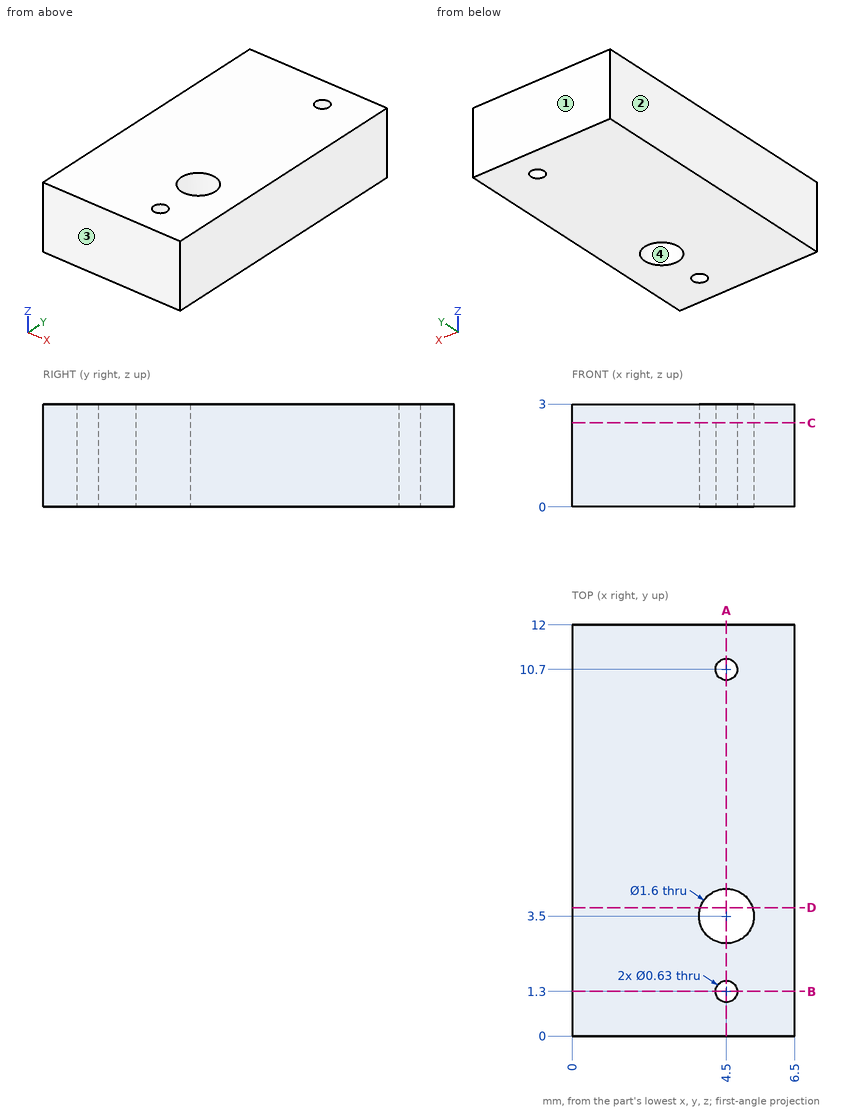
Part print with two shaded views. Sizes in mm from the minimum x, y, z corner. Coordinates: 2 decimals unless noted, no trailing zeros. Write each loop counter-clockwise with the first axis right and the second up, starting at its lowest first coordinate (ties: lowest second). Pieces come first, ordered by that corner, then holes.
(1) Cut at D-D on y = 3.75. List the corners of the cut face in (x, z).
(2) Drill centre lines: line 1 (Y direction, x = 4.5, z = 0.95) (3 decimals); line 2 (X direction, y = 3.5, z = 2.3); line 3 (Y direction, x = 4, z = 1.35). Where is each one in solid material? Low to high.
(3) Pin check, flat tip, straight feed: pin 1 Ø1.5 at (x, y) = (3, 6.5) entering from -Z. Stop position of the tip, or through.
(4) Mould opens along Y. For the marked faces 1, 2, 3 and 4 say: pulls with the +Y half, pulls with the -Y half, needs draft (parallel to the pull), parting line crosses it, or undercut.
(5) Cut at B-B on y = 1.3. List the corners of the cut face in (x, z) (3 decimals).
(6) Cut at C-C on z = 2.45. List the corners of the cut face in (x, y) (3 decimals), and give its area (3 significant figures).
(7) Cut at A-A on x = 4.5. List the corners of the cut face in (y, z) (3 decimals), and give its area (3 significant figures).
Working result:
1. outline: (0, 0) - (3.74, 0) - (3.74, 3) - (0, 3) - close; (5.26, 0) - (6.5, 0) - (6.5, 3) - (5.26, 3) - close
2. line 1: y = 0 to 0.985, 1.615 to 2.7, 4.3 to 10.385, 11.015 to 12
2. line 2: x = 0 to 3.7, 5.3 to 6.5
2. line 3: y = 0 to 2.88, 4.12 to 12
3. pin 1: stops at z = 0
4. face 1: pulls with the +Y half
4. face 2: needs draft
4. face 3: pulls with the -Y half
4. face 4: undercut
5. outline: (0, 0) - (4.185, 0) - (4.185, 3) - (0, 3) - close; (4.815, 0) - (6.5, 0) - (6.5, 3) - (4.815, 3) - close
6. outline: (0, 0) - (6.5, 0) - (6.5, 12) - (0, 12) - close; hole circle Ø1.6 at (4.5, 3.5); hole circle Ø0.63 at (4.5, 1.3); hole circle Ø0.63 at (4.5, 10.7)
6. area: 75.4 mm2
7. outline: (0, 0) - (0.985, 0) - (0.985, 3) - (0, 3) - close; (1.615, 0) - (2.7, 0) - (2.7, 3) - (1.615, 3) - close; (4.3, 0) - (10.385, 0) - (10.385, 3) - (4.3, 3) - close; (11.015, 0) - (12, 0) - (12, 3) - (11.015, 3) - close
7. area: 27.4 mm2
